Geometry check sheet. Reference: the model listing, model coordinates, mm. Round coordinates to 2 decimals unless told otherwise and drop trailing zeros. Loops run counter-clockwise (first coordinate to the right, second up) from the corner with the lowest first, then second, coordinate; pieces in that order, holes last.
```python
from build123d import *

# Parameters (mm, degrees)
SKETCH1_R               = 10
SKETCH1_R_2             = 5
BOSS_EXTRUDE1_DEPTH     = 338.5
CUT_EXTRUDE1_DEPTH      = 339.795292175
CUT_EXTRUDE1_DEPTH_BACK = 339.795292175
SKETCH2_R               = 2.5


with BuildPart() as part:
    # Sketch1 → Boss-Extrude1 (new, symmetric)
    with BuildSketch(Plane.XY):
        Circle(SKETCH1_R)
        Circle(SKETCH1_R_2, mode=Mode.SUBTRACT)
    extrude(amount=BOSS_EXTRUDE1_DEPTH, both=True)

    # Sketch2 → Cut-Extrude1 (cut, two sides: drawn at the far end of the back side and taken through both)
    with BuildSketch(Plane(origin=(0, 0, 0), x_dir=(1, 0, 0), z_dir=(0, 1, 0)).offset(-CUT_EXTRUDE1_DEPTH_BACK)):
        with Locations(Location((0, -328.5, 0), (0, 0, 270))):
            Circle(SKETCH2_R)
        with Locations(Location((0, 328.5, 0), (0, 0, 270))):
            Circle(SKETCH2_R)
    extrude(amount=CUT_EXTRUDE1_DEPTH + CUT_EXTRUDE1_DEPTH_BACK, mode=Mode.SUBTRACT)


solid = part.part
```
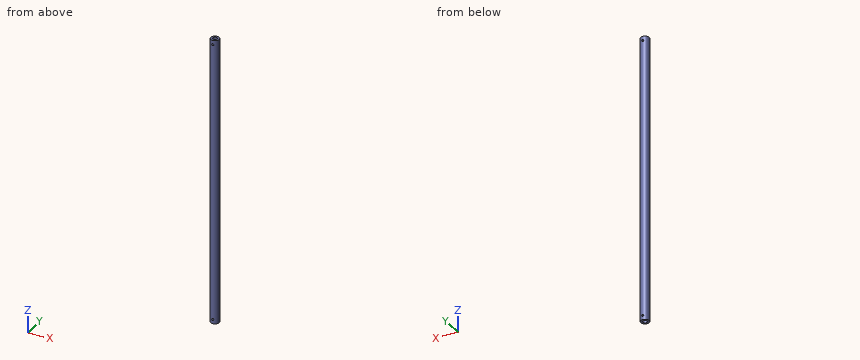
1) Gauge pin test, flat ends, axial feed: pin 1 (6.5 mm diameter, centred on x = 0, z = 328.5, fed in from -Y); pin 2 (8 mm diameter, centred on x = 7, z = -256.5, fed in from -Y); pin 3 (2 mm diameter, centred on x = -6, z = -139.5, fed in from +Y); pin 4 (1.5 mm diameter, centred on x = 3, z = 87.5, fed in from -Y). Record the tip position at first contact, or that the pin passes through.
Report:
pin 1: stops at y = -10
pin 2: stops at y = -9.54
pin 3: stops at y = 8.66
pin 4: stops at y = -9.74
2) Sectioned sample at B-B, the plane z = 97. Record the cut outline in (x, y), then the cut area to 3 significant figures.
Report:
outline: circle Ø20 at (0, 0); hole circle Ø10 at (0, 0)
area: 236 mm2
3) Sectioned sample at A-A, the plane y = 0. Record the cut outline in (x, z).
Report:
outline: (-10, -338.5) - (-5, -338.5) - (-5, 338.5) - (-10, 338.5) - close; (5, -338.5) - (10, -338.5) - (10, 338.5) - (5, 338.5) - close
4) Scan lines: line 1 along Z through (x, y) = (0, -7.3); line 2 along Y through (x, z) = (0, -111.5); line 3 along Z through (x, y) = (-1.75, -6.75). Record each from-to range of solid material in increasing order.
Report:
line 1: z = -338.5 to -331, -326 to 326, 331 to 338.5
line 2: y = -10 to -5, 5 to 10
line 3: z = -338.5 to -330.29, -326.71 to 326.71, 330.29 to 338.5
